```python
from build123d import *

# Parameters (mm, degrees)
MODEL_R             = 2.5
MODEL_R_2           = 2.05
MODEL_W             = 40
MODEL_H             = 24
BOSS_EXTRUDE1_DEPTH = 12


with BuildPart() as part:
    # Model → Boss-Extrude1 (new body)
    with BuildSketch(Plane.XY):
        Polygon((5, 275), (0, 270), (0, 5), (5, 0), (125, 0), (130, 5), (130, 270), (125, 275), align=None)
        with Locations((16.49, 6.5)):
            Circle(MODEL_R, mode=Mode.SUBTRACT)
        with Locations((48.83, 6.5)):
            Circle(MODEL_R, mode=Mode.SUBTRACT)
        with Locations((81.17, 6.5)):
            Circle(MODEL_R, mode=Mode.SUBTRACT)
        with Locations((113.51, 6.5)):
            Circle(MODEL_R, mode=Mode.SUBTRACT)
        with Locations((29, 128.5)):
            Circle(MODEL_R_2, mode=Mode.SUBTRACT)
        with Locations((65, 128.5)):
            Circle(MODEL_R_2, mode=Mode.SUBTRACT)
        with Locations((101, 128.5)):
            Circle(MODEL_R_2, mode=Mode.SUBTRACT)
        with Locations((101, 93.5)):
            Circle(MODEL_R_2, mode=Mode.SUBTRACT)
        with Locations((65, 93.5)):
            Circle(MODEL_R_2, mode=Mode.SUBTRACT)
        with Locations((29, 93.5)):
            Circle(MODEL_R_2, mode=Mode.SUBTRACT)
        with Locations((29, 267.5)):
            Circle(MODEL_R_2, mode=Mode.SUBTRACT)
        with Locations((65, 267.5)):
            Circle(MODEL_R_2, mode=Mode.SUBTRACT)
        with Locations((101, 267.5)):
            Circle(MODEL_R_2, mode=Mode.SUBTRACT)
        with Locations((101, 232.5)):
            Circle(MODEL_R_2, mode=Mode.SUBTRACT)
        with Locations((65, 232.5)):
            Circle(MODEL_R_2, mode=Mode.SUBTRACT)
        with Locations((29, 232.5)):
            Circle(MODEL_R_2, mode=Mode.SUBTRACT)
        with Locations((65, 111)):
            Rectangle(MODEL_W, MODEL_H, mode=Mode.SUBTRACT)
        with BuildLine():
            Line((13.99, 163.82), (13.99, 160.82))
            ThreePointArc((13.99, 160.82), (16.49, 158.32), (18.99, 160.82))
            Line((18.99, 160.82), (18.99, 163.82))
            ThreePointArc((18.99, 163.82), (16.49, 166.32), (13.99, 163.82))
        make_face(mode=Mode.SUBTRACT)
        with BuildLine():
            Line((46.33, 163.82), (46.33, 160.82))
            ThreePointArc((46.33, 160.82), (48.83, 158.32), (51.33, 160.82))
            Line((51.33, 160.82), (51.33, 163.82))
            ThreePointArc((51.33, 163.82), (48.83, 166.32), (46.33, 163.82))
        make_face(mode=Mode.SUBTRACT)
        with BuildLine():
            Line((78.67, 163.82), (78.67, 160.82))
            ThreePointArc((78.67, 160.82), (81.17, 158.32), (83.67, 160.82))
            Line((83.67, 160.82), (83.67, 163.82))
            ThreePointArc((83.67, 163.82), (81.17, 166.32), (78.67, 163.82))
        make_face(mode=Mode.SUBTRACT)
        with BuildLine():
            Line((111.01, 163.82), (111.01, 160.82))
            ThreePointArc((111.01, 160.82), (113.51, 158.32), (116.01, 160.82))
            Line((116.01, 160.82), (116.01, 163.82))
            ThreePointArc((116.01, 163.82), (113.51, 166.32), (111.01, 163.82))
        make_face(mode=Mode.SUBTRACT)
        with BuildLine():
            Line((13.99, 217), (13.99, 214))
            ThreePointArc((13.99, 214), (16.49, 211.5), (18.99, 214))
            Line((18.99, 214), (18.99, 217))
            ThreePointArc((18.99, 217), (16.49, 219.5), (13.99, 217))
        make_face(mode=Mode.SUBTRACT)
        with BuildLine():
            Line((51.33, 214), (51.33, 217))
            ThreePointArc((51.33, 217), (48.83, 219.5), (46.33, 217))
            Line((46.33, 217), (46.33, 214))
            ThreePointArc((46.33, 214), (48.83, 211.5), (51.33, 214))
        make_face(mode=Mode.SUBTRACT)
        with BuildLine():
            Line((83.67, 214), (83.67, 217))
            ThreePointArc((83.67, 217), (81.17, 219.5), (78.67, 217))
            Line((78.67, 217), (78.67, 214))
            ThreePointArc((78.67, 214), (81.17, 211.5), (83.67, 214))
        make_face(mode=Mode.SUBTRACT)
        with BuildLine():
            Line((116.01, 214), (116.01, 217))
            ThreePointArc((116.01, 217), (113.51, 219.5), (111.01, 217))
            Line((111.01, 217), (111.01, 214))
            ThreePointArc((111.01, 214), (113.51, 211.5), (116.01, 214))
        make_face(mode=Mode.SUBTRACT)
        with BuildLine():
            Line((18.99, 58.18), (18.99, 61.18))
            ThreePointArc((18.99, 61.18), (16.49, 63.68), (13.99, 61.18))
            Line((13.99, 61.18), (13.99, 58.18))
            ThreePointArc((13.99, 58.18), (16.49, 55.68), (18.99, 58.18))
        make_face(mode=Mode.SUBTRACT)
        with BuildLine():
            Line((51.33, 58.18), (51.33, 61.18))
            ThreePointArc((51.33, 61.18), (48.83, 63.68), (46.33, 61.18))
            Line((46.33, 61.18), (46.33, 58.18))
            ThreePointArc((46.33, 58.18), (48.83, 55.68), (51.33, 58.18))
        make_face(mode=Mode.SUBTRACT)
        with BuildLine():
            Line((83.67, 58.18), (83.67, 61.18))
            ThreePointArc((83.67, 61.18), (81.17, 63.68), (78.67, 61.18))
            Line((78.67, 61.18), (78.67, 58.18))
            ThreePointArc((78.67, 58.18), (81.17, 55.68), (83.67, 58.18))
        make_face(mode=Mode.SUBTRACT)
        with BuildLine():
            Line((116.01, 58.18), (116.01, 61.18))
            ThreePointArc((116.01, 61.18), (113.51, 63.68), (111.01, 61.18))
            Line((111.01, 61.18), (111.01, 58.18))
            ThreePointArc((111.01, 58.18), (113.51, 55.68), (116.01, 58.18))
        make_face(mode=Mode.SUBTRACT)
        with Locations((65, 250)):
            Rectangle(MODEL_W, MODEL_H, mode=Mode.SUBTRACT)
    extrude(amount=BOSS_EXTRUDE1_DEPTH)


solid = part.part
```
For this review, take the finished solid that the model builds, in its own axes (mm). A direction names the side the tool comes from. Coordinates: 2 decimals unless noted, no trailing zeros. Write each loop counter-clockwise with the first axis right and the second up, starting at its lowest first coordinate (ties: lowest second). Pieces come first, ordered by that corner, then holes.
(1) Tool access review of faces 1 (the face through (2, 3, 6)), 2 (the face through (48.78, 158.32, 5.92)): name each direction out of +Z, -Z, +X, -X, +Y, -Y from which nothing blocks a thin tool from reaching the whole face with its end or side.
(2) The part is to be moulded in two halves that separate along Y. For faces 3 (the face through (45, 111, 6)), 4 (the face through (128, 272, 6)), 5 (the face through (127, 2, 6)), 6 (the face through (16.44, 158.32, 5.92)), say which applies: +Y half, -Y half, draft (parallel to the pull), parting line (faces both ways), or undercut.
(3) Add section B-B on x = 72. Give the boundary of the cut face in (y, z), then the cut area to 3 significant figures.
(4) Wall thickness on probe 1 along Y at (x, z) = (29, 5.5); probe 2 along X at (y, z) = (232.5, 3); probe 3 along X at (y, z) = (249, 11.75): over which ranges is each line inside the solid? List them lowest first.
(5) Add section A-A on x = 113.51. Give the boundary of the cut face in (y, z).
(6) Add section C-C on z = 6.25. Count the separate pieces of the cut face and the enclosed holes in it, then the cut area to 3 significant figures.
Answer sheet:
1. face 1: +Z, -Z, -X, -Y
1. face 2: +Z, -Z
2. face 3: undercut
2. face 4: +Y half
2. face 5: -Y half
2. face 6: undercut
3. outline: (0, 0) - (99, 0) - (99, 12) - (0, 12) - close; (123, 0) - (238, 0) - (238, 12) - (123, 12) - close; (262, 0) - (275, 0) - (275, 12) - (262, 12) - close
3. area: 2,720 mm2
4. probe 1: y = 0 to 91.45, 95.55 to 126.45, 130.55 to 230.45, 234.55 to 265.45, 269.55 to 275
4. probe 2: x = 0 to 26.95, 31.05 to 62.95, 67.05 to 98.95, 103.05 to 130
4. probe 3: x = 0 to 45, 85 to 130
5. outline: (0, 0) - (4, 0) - (4, 12) - (0, 12) - close; (9, 0) - (55.68, 0) - (55.68, 12) - (9, 12) - close; (63.68, 0) - (158.32, 0) - (158.32, 12) - (63.68, 12) - close; (166.32, 0) - (211.5, 0) - (211.5, 12) - (166.32, 12) - close; (219.5, 0) - (275, 0) - (275, 12) - (219.5, 12) - close
6. separate pieces: 1
6. enclosed holes: 30
6. area: 33,100 mm2
